```python
from build123d import *

# Parameters (mm, degrees)
SKETCH1_W           = 54
SKETCH1_H           = 43
BOSS_EXTRUDE1_DEPTH = 5
CUT_EXTRUDE1_REACH  = 36.875
SKETCH2_R           = 1.55
SKETCH2_R_2         = 11.25
SKETCH4_W           = 5
SKETCH4_H           = 43
BOSS_EXTRUDE2_DEPTH = 80
CUT_EXTRUDE2_REACH  = 104.972
SKETCH6_R           = 2
SKETCH6_R_2         = 4.1
SKETCH7_R           = 3.5
CUT_EXTRUDE3_DEPTH  = 3
FILLET1_R           = 20


with BuildPart() as part:
    # Sketch1 → Boss-Extrude1 (new body)
    with BuildSketch(Plane(origin=(0, 0, 0), x_dir=(0, 0, -1), z_dir=(1, 0, 0))):
        Rectangle(SKETCH1_W, SKETCH1_H)
    extrude(amount=BOSS_EXTRUDE1_DEPTH)

    # Sketch2 → Cut-Extrude1 (cut, up to next)
    with BuildSketch(Plane(origin=(5, 0, 0), x_dir=(0, 0, -1), z_dir=(1, 0, 0)), mode=Mode.PRIVATE) as cut_extrude1_sk1:
        with Locations((-15.5, 15.5)):
            Circle(SKETCH2_R)
    cut_extrude1_tool1 = extrude(cut_extrude1_sk1.sketch, amount=-CUT_EXTRUDE1_REACH, mode=Mode.PRIVATE) & part.part
    # Sketch2 → Cut-Extrude1 (cut, up to next)
    with BuildSketch(Plane(origin=(5, 0, 0), x_dir=(0, 0, -1), z_dir=(1, 0, 0)), mode=Mode.PRIVATE) as cut_extrude1_sk2:
        with Locations((15.5, 15.5)):
            Circle(SKETCH2_R)
    cut_extrude1_tool2 = extrude(cut_extrude1_sk2.sketch, amount=-CUT_EXTRUDE1_REACH, mode=Mode.PRIVATE) & part.part
    # Sketch2 → Cut-Extrude1 (cut, up to next)
    with BuildSketch(Plane(origin=(5, 0, 0), x_dir=(0, 0, -1), z_dir=(1, 0, 0)), mode=Mode.PRIVATE) as cut_extrude1_sk3:
        with Locations((15.5, -15.5)):
            Circle(SKETCH2_R)
    cut_extrude1_tool3 = extrude(cut_extrude1_sk3.sketch, amount=-CUT_EXTRUDE1_REACH, mode=Mode.PRIVATE) & part.part
    # Sketch2 → Cut-Extrude1 (cut, up to next)
    with BuildSketch(Plane(origin=(5, 0, 0), x_dir=(0, 0, -1), z_dir=(1, 0, 0)), mode=Mode.PRIVATE) as cut_extrude1_sk4:
        with Locations((-15.5, -15.5)):
            Circle(SKETCH2_R)
    cut_extrude1_tool4 = extrude(cut_extrude1_sk4.sketch, amount=-CUT_EXTRUDE1_REACH, mode=Mode.PRIVATE) & part.part
    # Sketch2 → Cut-Extrude1 (cut, up to next)
    with BuildSketch(Plane(origin=(5, 0, 0), x_dir=(0, 0, -1), z_dir=(1, 0, 0)), mode=Mode.PRIVATE) as cut_extrude1_sk5:
        Circle(SKETCH2_R_2)
    cut_extrude1_tool5 = extrude(cut_extrude1_sk5.sketch, amount=-CUT_EXTRUDE1_REACH, mode=Mode.PRIVATE) & part.part
    add(cut_extrude1_tool1.solids().sort_by_distance((5, 15.5, 15.5))[0], mode=Mode.SUBTRACT)
    add(cut_extrude1_tool2.solids().sort_by_distance((5, 15.5, -15.5))[0], mode=Mode.SUBTRACT)
    add(cut_extrude1_tool3.solids().sort_by_distance((5, -15.5, -15.5))[0], mode=Mode.SUBTRACT)
    add(cut_extrude1_tool4.solids().sort_by_distance((5, -15.5, 15.5))[0], mode=Mode.SUBTRACT)
    add(cut_extrude1_tool5.solids().sort_by_distance((5, 0, 0))[0], mode=Mode.SUBTRACT)

    # Sketch4 → Boss-Extrude2 (add)
    with BuildSketch(Plane(origin=(5, 0, 0), x_dir=(0, 0, -1), z_dir=(1, 0, 0))):
        with Locations((-24.5, 0)):
            Rectangle(SKETCH4_W, SKETCH4_H)
    boss_extrude2 = extrude(amount=BOSS_EXTRUDE2_DEPTH)

    # Sketch6 → Cut-Extrude2 (cut, up to next)
    with BuildSketch(Plane.XY.offset(27), mode=Mode.PRIVATE) as cut_extrude2_sk1:
        with Locations((67, 12)):
            Circle(SKETCH6_R)
    cut_extrude2_tool1 = extrude(cut_extrude2_sk1.sketch, amount=-CUT_EXTRUDE2_REACH, mode=Mode.PRIVATE) & part.part
    # Sketch6 → Cut-Extrude2 (cut, up to next)
    with BuildSketch(Plane.XY.offset(27), mode=Mode.PRIVATE) as cut_extrude2_sk2:
        with Locations((79, 0)):
            Circle(SKETCH6_R)
    cut_extrude2_tool2 = extrude(cut_extrude2_sk2.sketch, amount=-CUT_EXTRUDE2_REACH, mode=Mode.PRIVATE) & part.part
    # Sketch6 → Cut-Extrude2 (cut, up to next)
    with BuildSketch(Plane.XY.offset(27), mode=Mode.PRIVATE) as cut_extrude2_sk3:
        with Locations((67, -12)):
            Circle(SKETCH6_R)
    cut_extrude2_tool3 = extrude(cut_extrude2_sk3.sketch, amount=-CUT_EXTRUDE2_REACH, mode=Mode.PRIVATE) & part.part
    # Sketch6 → Cut-Extrude2 (cut, up to next)
    with BuildSketch(Plane.XY.offset(27), mode=Mode.PRIVATE) as cut_extrude2_sk4:
        with Locations((55, 0)):
            Circle(SKETCH6_R)
    cut_extrude2_tool4 = extrude(cut_extrude2_sk4.sketch, amount=-CUT_EXTRUDE2_REACH, mode=Mode.PRIVATE) & part.part
    # Sketch6 → Cut-Extrude2 (cut, up to next)
    with BuildSketch(Plane.XY.offset(27), mode=Mode.PRIVATE) as cut_extrude2_sk5:
        with Locations((67, 0)):
            Circle(SKETCH6_R_2)
    cut_extrude2_tool5 = extrude(cut_extrude2_sk5.sketch, amount=-CUT_EXTRUDE2_REACH, mode=Mode.PRIVATE) & part.part
    cut_extrude2_1 = cut_extrude2_tool1.solids().sort_by_distance((67, 12, 27))[0]
    add(cut_extrude2_1, mode=Mode.SUBTRACT)
    cut_extrude2_2 = cut_extrude2_tool2.solids().sort_by_distance((79, 0, 27))[0]
    add(cut_extrude2_2, mode=Mode.SUBTRACT)
    cut_extrude2_3 = cut_extrude2_tool3.solids().sort_by_distance((67, -12, 27))[0]
    add(cut_extrude2_3, mode=Mode.SUBTRACT)
    cut_extrude2_4 = cut_extrude2_tool4.solids().sort_by_distance((55, 0, 27))[0]
    add(cut_extrude2_4, mode=Mode.SUBTRACT)
    cut_extrude2_5 = cut_extrude2_tool5.solids().sort_by_distance((67, 0, 27))[0]
    add(cut_extrude2_5, mode=Mode.SUBTRACT)
    cut_extrude2 = cut_extrude2_1 + cut_extrude2_2 + cut_extrude2_3 + cut_extrude2_4 + cut_extrude2_5  # Cut-Extrude2 as one shape, for the pattern or mirror that repeats it

    # Sketch7 → Cut-Extrude3 (cut)
    with BuildSketch(Plane.XY.offset(27)):
        with Locations((67, 12)):
            Circle(SKETCH7_R)
        with Locations((79, 0)):
            Circle(SKETCH7_R)
        with Locations((67, -12)):
            Circle(SKETCH7_R)
        with Locations((55, 0)):
            Circle(SKETCH7_R)
    cut_extrude3 = extrude(amount=-CUT_EXTRUDE3_DEPTH, mode=Mode.SUBTRACT)

    # Mirror2: Boss-Extrude2, Cut-Extrude2, Cut-Extrude3 across plane
    add(boss_extrude2.mirror(Plane.XY))
    add(cut_extrude2.mirror(Plane.XY), mode=Mode.SUBTRACT)
    add(cut_extrude3.mirror(Plane.XY), mode=Mode.SUBTRACT)

    # Fillet1
    fillet1_edges = [part.edges().sort_by_distance(p)[0] for p in [
        (85, -21.5, 24.5),
        (85, 21.5, 24.5),
        (85, 21.5, -24.5),
        (85, -21.5, -24.5),
    ]]
    fillet(fillet1_edges, radius=FILLET1_R)


solid = part.part
```
The model under review builds one solid part; all positions refer to its coordinate system, in mm. A direction names the side the tool comes from. Coordinates: 2 decimals unless noted, no trailing zeros. Order: outer loops, then holes, each group sorted by start corner. A loop starts at its lowest first (then second) coordinate and runs counter-clockwise, first axis right, second up. Notation, with made-up numbers: (-9, -30.5) -> (41, -30.5) arc R17 ccw to (41, -6.5) -> close; hole circle Ø5 at (-15.5, -25). An arc over 180 degrees is marked (long way). Answer in a Markdown table with one row per item. Add a question column.
Item 1: We need section D-D on z = 15.5. Write out the cut boundary in (x, y), plus the area to 3 significant figures.
Item 2: To check wall thickness, follow probe 1 along Z at (x, y) = (20, -19); probe 2 along Y at (x, z) = (55, -22.6); probe 3 along Y at (x, z) = (1.8, 15.5). State the ranges of each line that lie inside material, in increasing order.
Item 3: We need section C-C on y = 13. Write out the cut boundary in (x, z).
Item 4: Machinability: for faces 1 (the flat face through (44, 0, 22)), 2 (the flat face through (85, 0, 25)), 3 (the flat face through (69, 10, -24)), 4 (the flat face through (57, -2, 24)), which of the approach directions +Z, -Z, +X, -X, +Y, -Y give a long, thin tool a straight path to every point of the face, cutting with its end or side? Answer none if there is none.
Item 5: We need section B-B on z = 0. Write out the cut boundary in (x, y).
Item 6: Clearance check with flat-ended pins moving along their axes: pin 1 (5.5 mm diameter, centred on x = 67, y = -12, fed in from -Z); pin 2 (3.5 mm diameter, centred on x = 67, y = 12, fed in from +Z); pin 3 (5 mm diameter, centred on x = 79, y = 0, fed in from +Z); pin 4 (5 mm diameter, centred on y = 1, z = -21.5, fed in from +X). State where each tip first meets the part, or that it passes through.
Item 7: We need section A-A on x = 19. Write out the cut boundary in (y, z).
Item 8: Mouldability with a two-part tool opening along Y and no side actions: class faces 5 (the cylindrical face through (67, 14, -23)), 6 (the cylindrical face through (78.986, -15.797, 24.465)), 7 (the flat face through (81, -2, -24)), 8 (the flat face through (44, 0, -22)) as +Y half, -Y half, draft (parallel to the pull), parting line (faces both ways), or undercut.
Final values:
| question | item | result |
|---|---|---|
| 1 | outline | (0, -21.5) -> (5, -21.5) -> (5, -17.05) -> (0, -17.05) -> close; (0, -13.95) -> (5, -13.95) -> (5, 13.95) -> (0, 13.95) -> close; (0, 17.05) -> (5, 17.05) -> (5, 21.5) -> (0, 21.5) -> close |
| 1 | area | 184 mm2 |
| 2 | probe 1 | z = -27 to -22, 22 to 27 |
| 2 | probe 2 | y = -21.5 to -2, 2 to 21.5 |
| 2 | probe 3 | y = -21.5 to -17.05, -13.95 to 13.95, 17.05 to 21.5 |
| 3 | outline | (0, -27) -> (63.65, -27) -> (63.65, -24) -> (65.27, -24) -> (65.27, -22) -> (5, -22) -> (5, 22) -> (65.27, 22) -> (65.27, 24) -> (63.65, 24) -> (63.65, 27) -> (0, 27) -> close; (68.73, -24) -> (70.35, -24) -> (70.35, -27) -> (81.36, -27) -> (81.36, -22) -> (68.73, -22) -> close; (68.73, 22) -> (81.36, 22) -> (81.36, 27) -> (70.35, 27) -> (70.35, 24) -> (68.73, 24) -> close |
| 4 | face 1 | +X, +Y, -Y |
| 4 | face 2 | +Z, -Z, +X, +Y, -Y |
| 4 | face 3 | -Z |
| 4 | face 4 | +Z |
| 5 | outline | (0, -21.5) -> (5, -21.5) -> (5, -11.25) -> (0, -11.25) -> close; (0, 11.25) -> (5, 11.25) -> (5, 21.5) -> (0, 21.5) -> close |
| 6 | pin 1 | stops at z = -24 |
| 6 | pin 2 | passes through |
| 6 | pin 3 | stops at z = 24 |
| 6 | pin 4 | stops at x = 85 |
| 7 | outline | (-21.5, -27) -> (21.5, -27) -> (21.5, -22) -> (-21.5, -22) -> close; (-21.5, 22) -> (21.5, 22) -> (21.5, 27) -> (-21.5, 27) -> close |
| 8 | face 5 | undercut |
| 8 | face 6 | -Y half |
| 8 | face 7 | undercut |
| 8 | face 8 | draft |
